from build123d import *

# Parameters (mm, degrees)
ESTRUSIONE_ESTRUSIONE1_DEPTH = 4


with BuildPart() as part:
    # Schizzo1 → Estrusione-Estrusione1 (new body)
    with BuildSketch(Plane.XY):
        with BuildLine():
            Line((2, -11), (-2, -11))
            Line((-2, -11), (-2, -7))
            Line((-2, -7), (-12, -7))
            Line((-12, -7), (-26.333851616, 0.166925808))
            ThreePointArc((-26.333851616, 0.166925808), (-33.031566385, -0.74045287), (-34.635108255, -7.306377987))
            Line((-34.635108255, -7.306377987), (-29.5, -21))
            Line((-29.5, -21), (-28.5, -35))
            Line((-28.5, -35), (-29, -39))
            Line((-29, -39), (-29, -43))
            Line((-29, -43), (-27, -45))
            Line((-27, -45), (-27, -43))
            Line((-27, -43), (-23, -43))
            Line((-23, -43), (-23, -47.5))
            add(Edge.make_bspline(
                [(-23, -47.5), (-20.041371852, -48.760160273), (-17, -49)],
                knots=[0, 0, 0, 0.506712619, 0.506712619, 0.506712619], degree=2))
            Line((-17, -49), (-14.122054723, -49))
            add(Edge.make_bspline(
                [(-14.122054723, -49), (-12.571510592, -48.87926972), (-11, -48.5)],
                knots=[0.744931513, 0.744931513, 0.744931513, 1, 1, 1], degree=2))
            Line((-11, -48.5), (-11, -24))
            Line((-11, -24), (11, -24))
            Line((11, -24), (11, -48.5))
            add(Edge.make_bspline(
                [(11, -48.5), (12.571510592, -48.87926972), (14.122054723, -49)],
                knots=[0, 0, 0, 0.255068487, 0.255068487, 0.255068487], degree=2))
            Line((14.122054723, -49), (17, -49))
            add(Edge.make_bspline(
                [(17, -49), (20.041371852, -48.760160273), (23, -47.5)],
                knots=[0.493287381, 0.493287381, 0.493287381, 1, 1, 1], degree=2))
            Line((23, -47.5), (23, -43))
            Line((23, -43), (27, -43))
            Line((27, -43), (27, -45))
            Line((27, -45), (29, -43))
            Line((29, -43), (29, -39))
            Line((29, -39), (28.5, -35))
            Line((28.5, -35), (29.5, -21))
            Line((29.5, -21), (34.635108255, -7.306377987))
            ThreePointArc((34.635108255, -7.306377987), (33.031566385, -0.74045287), (26.333851616, 0.166925808))
            Line((26.333851616, 0.166925808), (12, -7))
            Line((12, -7), (2, -7))
            Line((2, -7), (2, -11))
        make_face()
        with BuildLine():
            ThreePointArc((24.854524092, -19.147929512), (20.47953862, -14.565955254), (15.276187318, -10.952076285))
            Line((15.276187318, -10.952076285), (26.292228197, -5.444055845))
            ThreePointArc((26.292228197, -5.444055845), (28.524799786, -5.746515405), (29.059313743, -7.935157111))
            Line((29.059313743, -7.935157111), (24.854524092, -19.147929512))
        make_face(mode=Mode.SUBTRACT)
        with BuildLine():
            ThreePointArc((-29.059313743, -7.935157111), (-28.524799786, -5.746515405), (-26.292228197, -5.444055845))
            Line((-26.292228197, -5.444055845), (-15.276187318, -10.952076285))
            ThreePointArc((-15.276187318, -10.952076285), (-20.47953862, -14.565955254), (-24.854524092, -19.147929512))
            Line((-24.854524092, -19.147929512), (-29.059313743, -7.935157111))
        make_face(mode=Mode.SUBTRACT)
    extrude(amount=ESTRUSIONE_ESTRUSIONE1_DEPTH)


solid = part.part
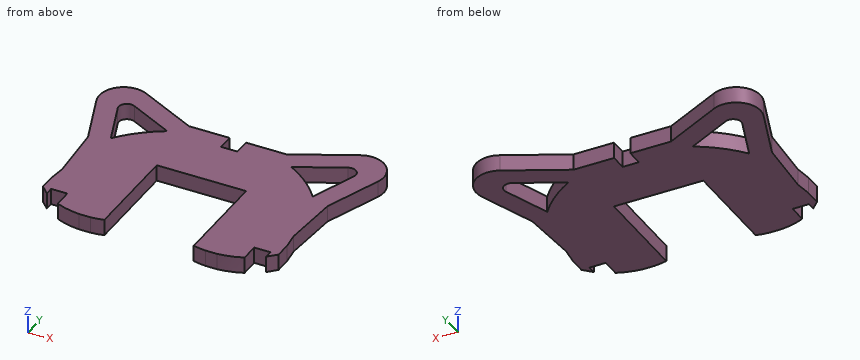
Work out the finished part from the listing and answer in its coordinate system (mm). Give positions to 0.01 mm unless a question says otherwise; leave off trailing zeros. Order: outer loops, then holes, each group sorted by start corner. A loop starts at its lowest first (then second) coordinate and runs counter-clockwise, first axis right, second up. Notation, with made-up numbers: (76.25, 87.5) -> (123.25, 87.5) arc R35 ccw to (123.25, 124.5) -> close; hole circle Ø6 at (-13.5, -24). An arc over 180 degrees is marked (long way). Answer as a JSON object with one key per item and string values. Group by question number.
1. Consider line 1 along X through (y, z) = (-46, 2.55); line 2 along X through (y, z) = (-39, 2.55); line 3 along X through (y, z) = (-12, 1.6) (3 decimals). Determine where each line is inside the solid, lowest interval first. Write a range as [from, to].
2. Section C-C on z = 1.8 is taken. Count the separate pieces of the cut face and the enclosed holes in it, plus the area to 3 significant figures.
3. Section D-D on x = -3.5 is taken. Determine the outline of the cut face in (y, z), plus the area to 3 significant figures.
4. Section A-A on y = -31.5 is taken. Determine the outline of the cut face in (x, z).
5. Section B-B on y = -9.5 is taken. Determine the outline of the cut face in (x, z), plus the area to 3 significant figures.
6. Flat-ended cylindrical pins translate along their axes: pin 1 Ø0.6 at (y, z) = (-44.5, 2) entering from +X; pin 2 Ø2 at (y, z) = (-34.5, 2.5) entering from +X; pin 3 Ø1.2 at (x, z) = (-0.5, 2) entering from +Y. Find the tip coordinate at first contact, or state that the pin passes through.
Result sheet:
{
 "1": {"line 1": "x = [-23, -11], [11, 23]", "line 2": "x = [-29, -11], [11, 29]", "line 3": "x = [-32.875, -27.535], [-17.029, 17.029], [27.535, 32.875]"},
 "2": {"separate pieces": "1", "enclosed holes": "2", "area": "1,920 mm^2"},
 "3": {"outline": "(-24, 0) -> (-7, 0) -> (-7, 4) -> (-24, 4) -> close", "area": "68.0 mm^2"},
 "4": {"outline": "(-28.75, 0) -> (-11, 0) -> (-11, 4) -> (-28.75, 4) -> close; (11, 0) -> (28.75, 0) -> (28.75, 4) -> (11, 4) -> close"},
 "5": {"outline": "(-33.81, 0) -> (-28.47, 0) -> (-28.47, 4) -> (-33.81, 4) -> close; (-18.18, 0) -> (-2, 0) -> (-2, 4) -> (-18.18, 4) -> close; (2, 0) -> (18.18, 0) -> (18.18, 4) -> (2, 4) -> close; (28.47, 0) -> (33.81, 0) -> (33.81, 4) -> (28.47, 4) -> close", "area": "172 mm^2"},
 "6": {"pin 1": "stops at x = 27.8", "pin 2": "stops at x = 28.61", "pin 3": "stops at y = -11"}
}
